Here's how the part is built. I have some questions about the finished solid (model axes, mm). Give positions to 0.01 mm unless a question says otherwise; leave off trailing zeros. Order: outer loops, then holes, each group sorted by start corner. A loop starts at its lowest first (then second) coordinate and runs counter-clockwise, first axis right, second up. Notation, with made-up numbers: M 76.25,63.25 L 113.25,63.25 A20 ccw 113.25,88.25 Z; hole C 55,8.25 d9. An arc over 180 degrees is marked long. One line per item, written item: value. Start each with the question number.
Autodesk Fusion 360 part; units mm, degrees
sketch "Sketch1" plane through (0, 0, 0) normal (0, 0, 1) x (1, 0, 0)
  line L0 (0, 0) -> (-25, 0)
  line L1 (-25, 0) -> (-25, 48)
  line L2 (-25, 48) -> (-23, 48)
  line L3 (-23, 48) -> (-23, 2)
  line L4 (-23, 2) -> (0, 2)
  line L5 (0, 2) -> (0, 0)
  dimension "d1" = 2
  dimension "d2" = 23
  dimension "d3" = 25
  dimension "d35" = 2
extrude "Extrude1" add sketch "Sketch1" along normal blind 68
sketch "Sketch2" plane through (-25, 0, 0) normal (-1, 0, 0) x (0, -1, 0)
  line L0 (-48, 0) -> (0, 0)
  line L1 (0, 0) -> (0, 68)
  line L2 (0, 68) -> (-48, 68)
  line L3 (-48, 68) -> (-48, 0)
  circle A0 centre (-6, 52.65) radius 1.75
  dimension "d8" = 3.5
  dimension "d9" = 15.35
  dimension "d10" = 6
extrude "Extrude2" cut sketch "Sketch2" against normal blind 15 contours A0
pattern_linear "R-Pattern1" count 1 spacing 0 along (0, 1, 0) count 2 spacing 37.3 along (0, 0, -1) of "Extrude2"
sketch "Sketch3" plane through (-25, 0, 0) normal (-1, 0, 0) x (0, -1, 0)
  circle A0 centre (-6, 15.35) radius 1.75
  circle A1 centre (-6, 52.65) radius 1.75
  line L0 (-48, 0) -> (0, 0)
  line L1 (0, 0) -> (0, 68)
  line L2 (0, 68) -> (-48, 68)
  line L3 (-48, 68) -> (-48, 0)
  circle A2 centre (-43.3, 52.65) radius 1.75
  dimension "d17" = 3.5
  dimension "d18" = 15.35
  dimension "d19" = 37.3
extrude "Extrude3" cut sketch "Sketch3" against normal blind 10 contours A2
pattern_linear "R-Pattern2" count 2 spacing 37.3 along (0, 0, -1) of "Extrude3"
sketch "Sketch4" plane through (0, 0, 0) normal (0, -1, 0) x (1, 0, 0)
  line L0 (-25, 0) -> (0, 0)
  line L1 (0, 0) -> (0, 68)
  line L2 (0, 68) -> (-25, 68)
  line L3 (-25, 68) -> (-25, 0)
  circle A0 centre (-6, 60) radius 1.475
  dimension "d26" = 2.95
  dimension "d27" = 8
  dimension "d28" = 6
extrude "Extrude4" cut sketch "Sketch4" against normal blind 6 contours A0
pattern_linear "R-Pattern3" count 3 spacing 26 along (0, 0, -1) of "Extrude4"
pattern_linear "R-Pattern4" count 2 spacing 10 along (0, 0, 1) of "R-Pattern2", "R-Pattern1", "Extrude3", "Extrude2"
pattern_linear "R-Pattern5" count 2 spacing 10 along (0, 0, -1) of "Extrude3", "Extrude2", "R-Pattern2", "R-Pattern1"
Item 1: Will these pins go through, and if not, where does the flat tip stop? P1, Ø1.5, axis at x = -14, z = 40, coming from the +Y side; P2, Ø4, axis at y = 6, z = 25.35, coming from the +X side.
Item 2: We'd pull the mould along Y, two halves only. Please class faces 1 (the face through (-7.474, 0.986, 8.065)), 2 (the face through (-24, 48, 34)), 3 (the face through (-24.01, 5.19, 23.8)): +Y half, -Y half, draft (parallel to the pull), parting line (faces both ways), or undercut.
Item 3: Please list where these lines run through material, in increasing order: probe 1 along Y at (x, z) = (-8.5, 57.5); probe 2 along X at (y, z) = (30.5, 38). Write a range as [from, to].
Item 4: I want a section at A-A on y = 6. Write out the boundary of the cut face in (x, z).
Item 5: I want a section at C-C on z = 60. Write out the boundary of the cut face in (x, y) (3 decimals).
Item 6: I want a section at B-B on x = -6. Write out the boundary of the cut face in (y, z) (3 decimals).
Item 7: I want a section at D-D on z = 40. Write out the boundary of the cut face in (x, y), plus the area to 3 significant figures.
Answer below:
1. P1: stops at y = 2
1. P2: stops at x = -23
2. face 1: draft
2. face 2: +Y half
2. face 3: undercut
3. probe 1: y = [0, 2]
3. probe 2: x = [-25, -23]
4. outline: M -25,0 L -23,0 L -23,3.6 L -25,3.6 Z; M -25,7.1 L -23,7.1 L -23,13.6 L -25,13.6 Z; M -25,17.1 L -23,17.1 L -23,23.6 L -25,23.6 Z; M -25,27.1 L -23,27.1 L -23,40.9 L -25,40.9 Z; M -25,44.4 L -23,44.4 L -23,50.9 L -25,50.9 Z; M -25,54.4 L -23,54.4 L -23,60.9 L -25,60.9 Z; M -25,64.4 L -23,64.4 L -23,68 L -25,68 Z
5. outline: M -25,0 L -7.475,0 L -7.475,2 L -23,2 L -23,48 L -25,48 Z; M -4.525,0 L 0,0 L 0,2 L -4.525,2 Z
6. outline: M 0,0 L 2,0 L 2,6.525 L 0,6.525 Z; M 0,9.475 L 2,9.475 L 2,32.525 L 0,32.525 Z; M 0,35.475 L 2,35.475 L 2,58.525 L 0,58.525 Z; M 0,61.475 L 2,61.475 L 2,68 L 0,68 Z
7. outline: M -25,0 L 0,0 L 0,2 L -23,2 L -23,48 L -25,48 Z
7. area: 142 mm²
